CAD build for the part. Positions are in the model's coordinates, mm. A direction names the side the tool comes from. Give positions to 0.01 mm unless a question says otherwise; leave off trailing zeros. Order: outer loops, then holes, each group sorted by start corner. A loop starts at its lowest first (then second) coordinate and runs counter-clockwise, first axis right, second up.
Item 1: Band-saw the part on B-B on z = 35. Give the cut face in (x, y).
Item 2: Flat gauge pins, fed straight in: P1, Ø10, axis at y = -63, z = 63.5, coming from the +X side; P2, Ø6, axis at y = -41.5, z = 55, coming from the +X side; P3, Ø10, axis at x = 28, y = -65, coming from the +Z side. Where does each tip first touch, or does it go through?
Item 3: Band-saw the part on C-C on x = 51.5. Give the cut face in (y, z).
Item 4: Band-saw the part on D-D on z = 53. Give the cut face in (x, y), plus the area to 3 significant figures.
Item 5: Which spindle directions (+Z, -Z, +X, -X, +Y, -Y) get a long thin tool onto all of the face, cutting with end or side? Do faces 1 (the flat face through (39.778, -50.444, 47.409)), 2 (the flat face through (-42.13, -50.44, 51.48)), 3 (the flat face through (-3, -38, -25.496)). Say none if no direction does.
Item 6: Wall check: L1, parallel to Y at x = 65, z = 48; L2, parallel to X at y = -34, z = 51.5; L3, parallel to Z at x = 54, y = -62.5. Give the ranges that are in metal, low to high.
Item 7: Band-saw the part on A-A on y = -56.5. Give the cut face in (x, z), plus the area to 3 significant figures.
```python
from build123d import *

# Parameters (mm, degrees)
F0_W     = 148.8501727581
F0_H     = 101.742612198
F1_DEPTH = 50.8
F3_DEPTH = 25.4
F5_DEPTH = 25.4


with BuildPart() as f1:
    # F0 (on Front) → F1 (new body)
    with BuildSketch(Plane.XZ):
        with Locations((-1.6997531056, 25.3749480471)):
            Rectangle(F0_W, F0_H)
    extrude(amount=F1_DEPTH)

    # F2 (on face) → F3 (cut)
    with BuildSketch(Plane.XZ.offset(50.8)):
        Polygon((-9.0788973585, 76.2462541461), (-76.1248394847, 76.2462541461), (-76.1248394847, 26.0104050889), align=None)
        Polygon((72.7253332734, 76.2462541461), (5.8954056378, 76.2462541461), (72.7253332734, 19.3677039224), align=None)
    extrude(amount=-F3_DEPTH, mode=Mode.SUBTRACT)

    # F1_face (on face) + F4 (on face) → F5 (join)
    with BuildSketch(Plane(origin=(-1.6997531056, -50.8, 25.3749480471), x_dir=(1, 0, 0), z_dir=(0, -1, 0))):
        Polygon((74.4250863791, -6.0072441247), (7.5951587435, 50.871306099), (-7.3791442529, 50.871306099), (-74.4250863791, 0.6354570418), (-74.4250863791, -50.871306099), (74.4250863791, -50.871306099), align=None)
    with BuildSketch(Plane.XZ.offset(50.8)):
        Polygon((72.7253332734, -25.4963580519), (72.7253332734, 19.3677039224), (5.8954056378, 76.2462541461), (-9.0788973585, 76.2462541461), (-76.1248394847, 26.0104050889), (-76.1248394847, -25.4963580519), align=None)
    extrude(amount=F5_DEPTH)


solid = f1.part
```
The answers:
1. outline: (-76.12, -25.4) - (-64.13, -25.4) - (-64.13, -76.2) - (54.36, -76.2) - (54.36, -25.4) - (72.73, -25.4) - (72.73, 0) - (-76.12, 0) - close
2. P1: stops at x = 26.75
2. P2: stops at x = 34.38
2. P3: stops at z = 61.69
3. outline: (-76.2, -25.5) - (0, -25.5) - (0, 76.25) - (-25.4, 76.25) - (-25.4, 37.43) - (-76.2, 37.43) - close
4. outline: (-76.12, -25.4) - (-40.1, -25.4) - (-40.1, -76.2) - (33.21, -76.2) - (33.21, -25.4) - (72.73, -25.4) - (72.73, 0) - (-76.12, 0) - close
4. area: 7,510 mm2
5. face 1: +Z, +X, -Y
5. face 2: +Z, -X, -Y
5. face 3: -Z, +X, -X, +Y, -Y
6. L1: y = -25.4 to 0
6. L2: x = -42.11 to 34.97
6. L3: z = -25.5 to 35.3
7. outline: (-76.12, -25.5) - (72.73, -25.5) - (72.73, 19.37) - (5.9, 76.25) - (-9.08, 76.25) - (-76.12, 26.01) - close
7. area: 11,600 mm2
